from build123d import *

# Parameters (mm, degrees)
SKETCH5_R                      = 26
BOSS_EXTRUDE3_DEPTH            = 13
SKETCH6_R                      = 24.9
BOSS_EXTRUDE4_DEPTH            = 7
M3_CLEARANCE_HOLE1_D           = 3.4
M3_CLEARANCE_HOLE1_CSINK_D     = 3.45
M3_CLEARANCE_HOLE1_CSINK_ANGLE = 90


with BuildPart() as part:
    # Sketch5 → Boss-Extrude3 (new body)
    with BuildSketch(Plane(origin=(0, 0, 0), x_dir=(-1, 0, 0), z_dir=(0, 1, 0))):
        with Locations(Location((0, 0, 0), (0, 0, 270))):
            Circle(SKETCH5_R)
    extrude(amount=BOSS_EXTRUDE3_DEPTH)

    # Sketch6 → Boss-Extrude4 (add)
    with BuildSketch(Plane(origin=(0, 13, 0), x_dir=(-1, 0, 0), z_dir=(0, 1, 0))):
        with Locations(Location((0, 0, 0), (0, 0, 90))):
            Circle(SKETCH6_R)
    extrude(amount=BOSS_EXTRUDE4_DEPTH)

    # M3 Clearance Hole1 (through all)
    with Locations(Plane(origin=(0, 20, 0), x_dir=(-1, 0, 0), z_dir=(0, 1, 0))):
        with Locations((-6.318103468, -15.253251082), (-10.050651193, 13.098263648), (16.368754661, 2.154987434)):
            CounterSinkHole(M3_CLEARANCE_HOLE1_D / 2, M3_CLEARANCE_HOLE1_CSINK_D / 2, counter_sink_angle=M3_CLEARANCE_HOLE1_CSINK_ANGLE)


solid = part.part
The model under review builds one solid part; all positions refer to its coordinate system, in mm. Round coordinates to 2 decimals unless told otherwise and drop trailing zeros. Order: outer loops, then holes, each group sorted by start corner. A loop starts at its lowest first (then second) coordinate and runs counter-clockwise, first axis right, second up. Notation, with made-up numbers: (78, 3.5) -> (82, 3.5) arc R27 ccw to (82, 34.5) -> close; hole circle Ø4 at (76, 23). An arc over 180 degrees is marked (long way). Use CSV: the item, a comma, the result in double quotes. Start each with the question number.
(1) Consider section A-A on z = 22. Write out the cut boundary in (x, y), and give its area (3 significant figures).
(2) Consider section D-D on y = 6.5. Write out the cut boundary in (x, z).
(3) Consider section B-B on x = 15. Write out the cut boundary in (y, z), and give its area (3 significant figures).
(4) Mouldability with a two-part tool opening along X and no side actions: class faces 1 (the face through (6.097, 9.848, -13.568)), 2 (the face through (-15.15, 16.45, -19.76)), 3 (the face through (2, 13, -25)) as pulls with the +X half, pulls with the -X half, needs draft (parallel to the pull), parting line crosses it, or undercut.
(5) Wall thickness on probe 1 along Y at (x, z) = (-6, 24.5); probe 2 along X at (y, z) = (10.5, 3.5); probe 3 along X at (y, z) = (12.5, 1.5): over which ranges is each line inside the solid? List them lowest first. Write a range as from..to.
(6) Insertion check: pin 1 (1 mm diameter, centred on y = 14.5, z = -16, fed in from -X); pin 2 (8 mm diameter, centred on x = 18.5, y = 16, fed in from +Z); pin 3 (10 mm diameter, centred on y = 6, z = -17.5, fed in from +X). Each pin has a flat end and moves straight along its axis. Give the tip position at first contact, or say it passes through.
(7) Consider section C-C on y = 18.25. Write out the cut boundary in (x, z), and give its area (3 significant figures).
Responses:
1,outline,"(-13.86, 0) -> (13.86, 0) -> (13.86, 13) -> (11.66, 13) -> (11.66, 20) -> (-11.66, 20) -> (-11.66, 13) -> (-13.86, 13) -> close"
1,area,"524 mm²"
2,outline,"circle Ø52 at (0, 0); hole circle Ø3.4 at (-16.37, 2.15); hole circle Ø3.4 at (6.32, -15.25); hole circle Ø3.4 at (10.05, 13.1)"
3,outline,"(0, -21.24) -> (13, -21.24) -> (13, -19.87) -> (20, -19.87) -> (20, 19.87) -> (13, 19.87) -> (13, 21.24) -> (0, 21.24) -> close"
3,area,"830 mm²"
4,face 1,"undercut"
4,face 2,"parting line crosses it"
4,face 3,"needs draft"
5,probe 1,"0..13"
5,probe 2,"-25.76..-17.41, -15.33..25.76"
5,probe 3,"-25.96..-17.94, -14.8..25.96"
6,pin 1,"x = -19.49"
6,pin 2,"z = 20.61"
6,pin 3,"x = 22.8"
7,outline,"circle Ø49.8 at (0, 0); hole circle Ø3.4 at (-16.37, 2.15); hole circle Ø3.4 at (6.32, -15.25); hole circle Ø3.4 at (10.05, 13.1)"
7,area,"1,920 mm²"
